Build history of the part. All positions in model axes, mm. A direction names the side the tool comes from. Coordinates: 2 decimals unless noted, no trailing zeros. Write each loop counter-clockwise with the first axis right and the second up, starting at its lowest first coordinate (ties: lowest second). Pieces come first, ordered by that corner, then holes.
from build123d import *

# Parameters (mm, degrees)
SKETCH2_R          = 4.7625
SKETCH2_R_2        = 3.175
SKETCH11_W         = 4
SKETCH11_H         = 4.7625
CUT_EXTRUDE2_DEPTH = 8


with BuildPart() as part:
    # Sweep2: sweep along a path in Sketch4
    with BuildLine(Plane(origin=(0, 0, 0), x_dir=(0, 0, -1), z_dir=(1, 0, 0))) as sweep2_path:
        Line((8, 0), (8, 45))
        Line((8, 45), (168, 245))
        Line((168, 245), (237.282032303, 285))
    # Sketch2 → Sweep2 (sweep)
    with BuildSketch(Plane(origin=(0, 0, 0), x_dir=(1, 0, 0), z_dir=(0, 1, 0))):
        with Locations((0, 8)):
            Circle(SKETCH2_R)
        with Locations((0, 8)):
            Circle(SKETCH2_R_2, mode=Mode.SUBTRACT)
    sweep(path=sweep2_path.line, transition=Transition.RIGHT)

    # Sketch11 → Cut-Extrude2 (cut)
    with BuildSketch(Plane(origin=(0, 158.996133918, -275.389382153), x_dir=(1, 0, 0), z_dir=(0, 0.5, -0.866025404))):
        with Locations((0, -125.794973927)):
            Rectangle(SKETCH11_W, SKETCH11_H)
    extrude(amount=-CUT_EXTRUDE2_DEPTH, mode=Mode.SUBTRACT)


solid = part.part
(1) Flat gauge pins, fed straight in: P1, Ø3, axis at x = 3.5, z = -97, coming from the +Y side; P2, Ø1.5, axis at x = 3, y = 146.5, coming from the +Z side; P3, Ø5, axis at x = 2, z = -117.5, coming from the +Y side. Where does each tip first touch, or does it go through?
(2) 3-axis set-ups, long thin cutter, end or side, ignore diameter. For faces 3 (the cylindrical face through (2.2, 148.75, -85.59)), 4 (the cylindrical face through (-1.03, 23.66, -3.35)): which of +Z, -Z, +X, -X, +Y, -Y reach the whole face in a straight line?
(3) Slice it at A-A, the plane x = 0. List the corners of the cut face in (y, z) (1 decimal).
(4) Probe L1, parallel to X at y = 13.5, z = -8 (1 decimal); L2, parallel to Z at x = 0, y = 23 (1 decimal); L3, parallel to Y at x = -1.25, z = -198.5. List the from-to ranges inside material, lowest first.
(5) Two-plate mould, pull along X, no slides. Class faces 1 (the cylindrical face through (2.2, 268.7, -200.6)), 2 (the flat face through (2, 265, -210)): pulls with the +X half, pulls with the -X half, needs draft (parallel to the pull), parting line crosses it, or undercut.
Results:
1. P1: stops at y = 164.14
1. P2: stops at z = -83.56
1. P3: stops at y = 192.21
2. face 3: none
2. face 4: -Y
3. outline: (0, -12.8) - (43.3, -12.8) - (241.3, -171.2) - (261.9, -206.8) - (263.3, -206) - (242.5, -170.1) - (43.9, -11.2) - (0, -11.2) - close; (0, -4.8) - (46.1, -4.8) - (247.5, -165.9) - (287.7, -235.7) - (289.1, -234.9) - (248.7, -164.8) - (46.7, -3.2) - (0, -3.2) - close; (265.9, -213.7) - (280.9, -239.7) - (282.3, -238.9) - (267.3, -212.9) - close
4. L1: x = -4.8 to -3.2, 3.2 to 4.8
4. L2: z = -12.8 to -11.2, -4.8 to -3.2
4. L3: y = 257.3 to 259.24, 265.98 to 267.92
5. face 1: parting line crosses it
5. face 2: undercut
